Verification items for the finished model (mm, model axes). Coordinates: 2 decimals unless noted, no trailing zeros. Write each loop counter-clockwise with the first axis right and the second up, starting at its lowest first coordinate (ties: lowest second). Pieces come first, ordered by that corner, then holes. Notation, with made-up numbers: (31.25, 68.25) - (40.25, 68.25) arc R15 cw to (40.25, 91.25) - close; hole circle Ø11 at (-39, 50.5). An arc over 180 degrees is marked (long way). Use one line per item in the form item = value. Start each with the question number.
(1) Material ranges on line 1 (X direction, y = -3.6, z = -83); line 2 (X direction, y = -0.7, z = -8.5); line 3 (Z direction, x = 615, y = -1.7), recorded low to high. Write a range as [from, to].
(2) Gauge pin test, flat ends, axial feed: pin 1 Ø3 at (y, z) = (-4, -31.5) entering from +X; pin 2 Ø1.5 at (x, y) = (146, -1.5) entering from +Z; pin 3 Ø2 at (y, z) = (-4.5, -77) entering from -X. Record the tip position at first contact, or that the pin passes through.
(3) Sectioned sample at C-C (y = -1.65). Count the separate pieces of the cut face and the enclosed holes in it, and give its area (3 significant figures).
(4) Sectioned sample at B-B (x = 595). Record the cut outline in (y, z).
(5) Sectioned sample at A-A (z = -17). Record the cut outline in (x, y).
from build123d import *

# Parameters (mm, degrees)
F1_DEPTH = 6


with BuildPart() as f1:
    # F0 (on Front) → F1 (new body)
    with BuildSketch(Plane.XZ):
        Polygon((184, 0), (0, 0), (0, -35.21), (-5.8, -35.21), (-5.8, -37.21), (-3, -39.21), (-3, -49.21), (-5.8, -51.21), (-5.8, -53.21), (0, -53.21), (0, -103.23), (-5.8, -103.23), (-5.8, -105.23), (-3, -107.23), (-3, -117.23), (-5.8, -119.23), (-5.8, -121.23), (0, -121.23), (0, -144), (888, -144), (888, -121.23), (893.8, -121.23), (893.8, -119.23), (891, -117.23), (891, -107.23), (893.8, -105.23), (893.8, -103.23), (888, -103.23), (888, -53.21), (893.8, -53.21), (893.8, -51.21), (891, -49.21), (891, -39.21), (893.8, -37.21), (893.8, -35.21), (888, -35.21), (888, 0), (704, 0), (704, -72.01), (697.99, -72.01), (697.99, 0), (675, 0), (675, 5.8), (673, 5.8), (671, 3), (661, 3), (659, 5.8), (657, 5.8), (657, 0), (538.8, 0), (538.8, -72.01), (532.79, -72.01), (532.79, 0), (453, 0), (453, 5.8), (451, 5.8), (449, 3), (439, 3), (437, 5.8), (435, 5.8), (435, 0), (355.21, 0), (355.21, -72.01), (349.2, -72.01), (349.2, 0), (231, 0), (231, 5.8), (229, 5.8), (227, 3), (217, 3), (215, 5.8), (213, 5.8), (213, 0), (190.01, 0), (190.01, -72.01), (184, -72.01), align=None)
        with BuildLine():
            ThreePointArc((30, -35), (31.464466, -31.464466), (35, -30))
            Line((35, -30), (149, -30))
            ThreePointArc((149, -30), (152.535534, -31.464466), (154, -35))
            Line((154, -35), (154, -109))
            ThreePointArc((154, -109), (152.535534, -112.535534), (149, -114))
            Line((149, -114), (35, -114))
            ThreePointArc((35, -114), (31.464466, -112.535534), (30, -109))
            Line((30, -109), (30, -35))
        make_face(mode=Mode.SUBTRACT)
        with BuildLine():
            Line((220.01, -109), (220.01, -35))
            ThreePointArc((220.01, -35), (221.474466, -31.464466), (225.01, -30))
            Line((225.01, -30), (314.2, -30))
            ThreePointArc((314.2, -30), (317.735534, -31.464466), (319.2, -35))
            Line((319.2, -35), (319.2, -109))
            ThreePointArc((319.2, -109), (317.735534, -112.535534), (314.2, -114))
            Line((314.2, -114), (225.01, -114))
            ThreePointArc((225.01, -114), (221.474466, -112.535534), (220.01, -109))
        make_face(mode=Mode.SUBTRACT)
        with BuildLine():
            ThreePointArc((385.21, -35), (386.674466, -31.464466), (390.21, -30))
            Line((390.21, -30), (497.79, -30))
            ThreePointArc((497.79, -30), (501.325534, -31.464466), (502.79, -35))
            Line((502.79, -35), (502.79, -109))
            ThreePointArc((502.79, -109), (501.325534, -112.535534), (497.79, -114))
            Line((497.79, -114), (390.21, -114))
            ThreePointArc((390.21, -114), (386.674466, -112.535534), (385.21, -109))
            Line((385.21, -109), (385.21, -35))
        make_face(mode=Mode.SUBTRACT)
        with BuildLine():
            ThreePointArc((568.8, -35), (570.264466, -31.464466), (573.8, -30))
            Line((573.8, -30), (662.99, -30))
            ThreePointArc((662.99, -30), (666.525534, -31.464466), (667.99, -35))
            Line((667.99, -35), (667.99, -109))
            ThreePointArc((667.99, -109), (666.525534, -112.535534), (662.99, -114))
            Line((662.99, -114), (573.8, -114))
            ThreePointArc((573.8, -114), (570.264466, -112.535534), (568.8, -109))
            Line((568.8, -109), (568.8, -35))
        make_face(mode=Mode.SUBTRACT)
        with BuildLine():
            ThreePointArc((734, -35), (735.464466, -31.464466), (739, -30))
            Line((739, -30), (853, -30))
            ThreePointArc((853, -30), (856.535534, -31.464466), (858, -35))
            Line((858, -35), (858, -109))
            ThreePointArc((858, -109), (856.535534, -112.535534), (853, -114))
            Line((853, -114), (739, -114))
            ThreePointArc((739, -114), (735.464466, -112.535534), (734, -109))
            Line((734, -109), (734, -35))
        make_face(mode=Mode.SUBTRACT)
    extrude(amount=F1_DEPTH)


solid = f1.part
Answers below:
q1.line_1 = [0, 30], [154, 220.01], [319.2, 385.21], [502.79, 568.8], [667.99, 734], [858, 888]
q1.line_2 = [0, 184], [190.01, 349.2], [355.21, 532.79], [538.8, 697.99], [704, 888]
q1.line_3 = [-144, -114], [-30, 0]
q2.pin_1 = 888
q2.pin_2 = 0
q2.pin_3 = 0
q3.separate_pieces = 1
q3.enclosed_holes = 5
q3.area = 79,400 mm2
q4.outline = (-6, -144) - (0, -144) - (0, -114) - (-6, -114) - close; (-6, -30) - (0, -30) - (0, 0) - (-6, 0) - close
q5.outline = (0, -6) - (184, -6) - (184, 0) - (0, 0) - close; (190.01, -6) - (349.2, -6) - (349.2, 0) - (190.01, 0) - close; (355.21, -6) - (532.79, -6) - (532.79, 0) - (355.21, 0) - close; (538.8, -6) - (697.99, -6) - (697.99, 0) - (538.8, 0) - close; (704, -6) - (888, -6) - (888, 0) - (704, 0) - close
